The model under review builds one solid part; all positions refer to its coordinate system, in mm. Face numbers are marked on the shaded views. A direction names the side the tool comes from. Round coordinates to 2 decimals unless told otherwise and drop trailing zeros. Order: outer loops, then holes, each group sorted by start corner. A loop starts at its lowest first (then second) coordinate and runs counter-clockwise, first axis right, second up. Notation, with made-up numbers: M 55,52.5 L 68,52.5 A32 ccw 68,81.5 Z; hole C 54,-9.75 d9. An arc over 180 degrees is marked long. One line per item, written item: value. Start each with the question number.
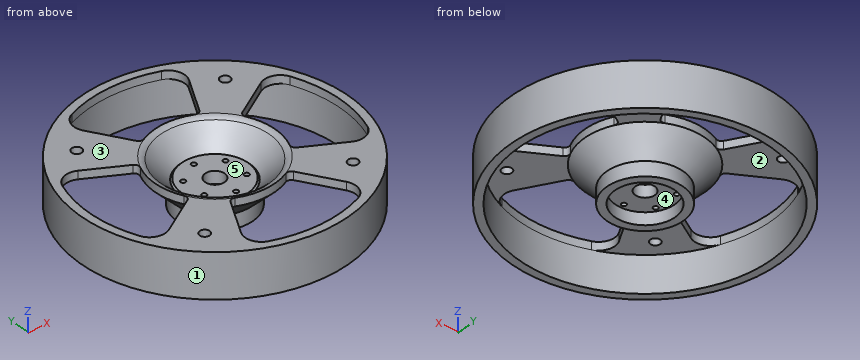
from build123d import *

# Parameters (mm, degrees)
EXTRUDE_1_DEPTH          = 20
EXTRUDE_1_DEPTH_BACK     = 7.5
SKETCH_1_R               = 82.5
SKETCH_1_R_2             = 80
EXTRUDE_3_DEPTH          = 7.5
EXTRUDE_3_DEPTH_BACK     = 7.5
SKETCH_3_R               = 21.5
CHAMFER_1_SIZE           = 1
SKETCH_4_R               = 18.5
CUT_EXTRUDE_1_DEPTH      = 7.5
SKETCH_5_R               = 1.5
CUT_EXTRUDE_2_DEPTH      = 7.5
SKETCH_6_R               = 6
CUT_EXTRUDE_3_DEPTH      = 7.5
SKETCH_9_R               = 3.1
CUT_EXTRUDE_4_DEPTH      = 119.822346
CUT_EXTRUDE_5_DEPTH      = 10
CUT_EXTRUDE_5_DEPTH_BACK = 119.822346


# Read off the part's stored shape, not the designer's step: the shell step
with BuildPart() as part:
    # Sketch 1 → Extrude 1 (new, two sides: drawn at the far end of the back side and taken through both)
    with BuildSketch(Plane.XY.offset(-EXTRUDE_1_DEPTH_BACK)):
        Circle(SKETCH_1_R)
        Circle(SKETCH_1_R_2, mode=Mode.SUBTRACT)
    extrude(amount=EXTRUDE_1_DEPTH + EXTRUDE_1_DEPTH_BACK)



with BuildPart() as body_2:
    # Sketch 3 → Extrude 3 (new, two sides: drawn at the far end of the back side and taken through both)
    with BuildSketch(Plane.XY.offset(-EXTRUDE_3_DEPTH_BACK)):
        Circle(SKETCH_3_R)
    extrude(amount=EXTRUDE_3_DEPTH + EXTRUDE_3_DEPTH_BACK)

    # Chamfer 1
    chamfer_1_edges = [body_2.edges().sort_by_distance(p)[0] for p in [
        (-21.5, 0, 7.5),
    ]]
    chamfer(chamfer_1_edges, length=CHAMFER_1_SIZE)

    # Sketch 4 → Cut-Extrude 1 (cut)
    with BuildSketch(Plane(origin=(0, 0, -7.5), x_dir=(-1, 0, 0), z_dir=(0, 0, -1))):
        Circle(SKETCH_4_R)
    extrude(amount=-CUT_EXTRUDE_1_DEPTH, mode=Mode.SUBTRACT)

    # Sketch 5 → Cut-Extrude 2 (cut)
    with BuildSketch(Plane.XY.offset(7.5)):
        with Locations((0, 15.5)):
            Circle(SKETCH_5_R)
        with Locations((13.423394, 7.75)):
            Circle(SKETCH_5_R)
        with Locations((13.423394, -7.75)):
            Circle(SKETCH_5_R)
        with Locations((0, -15.5)):
            Circle(SKETCH_5_R)
        with Locations((-13.423394, -7.75)):
            Circle(SKETCH_5_R)
        with Locations((-13.423394, 7.75)):
            Circle(SKETCH_5_R)
    extrude(amount=-CUT_EXTRUDE_2_DEPTH, mode=Mode.SUBTRACT)

    # Sketch 6 → Cut-Extrude 3 (cut)
    with BuildSketch(Plane.XY.offset(7.5)):
        Circle(SKETCH_6_R)
    extrude(amount=-CUT_EXTRUDE_3_DEPTH, mode=Mode.SUBTRACT)


with BuildPart() as part_1:
    add(part.part)

    add(body_2.part)  # Revolve 1 merges body 2
    # Sketch 8 → Revolve 1 (revolve)
    with BuildSketch(Plane(origin=(0, 0, 0), x_dir=(1, 0, 0), z_dir=(0, 1, 0)), mode=Mode.PRIVATE) as revolve_1_sk:
        with BuildLine():
            Line((-37.071068, -20), (-80, -20))
            Line((-80, -20), (-80, 0))
            Line((-80, 0), (-80, 0.5))
            Line((-80, 0.5), (-80, 7.5))
            Line((-80, 7.5), (-21.5, 7.5))
            Line((-21.5, 7.5), (-21.5, -6.5))
            Line((-21.5, -6.5), (-33.535534, -18.535534))
            ThreePointArc((-33.535534, -18.535534), (-35.157651, -19.619398), (-37.071068, -20))
        make_face()
    revolve(revolve_1_sk.sketch.rotate(Axis((0, 0, 0), (0, 0, -1)), 180), axis=Axis((0, 0, 0), (0, 0, -1)))

    # Shell 1 outline → Shell 1 (revolve, cut)
    with BuildSketch(Plane.XZ):
        Polygon((37.071068, 15), (23.5, 1.428932), (23.5, -7.5), (77.5, -7.5), (77.5, 15), align=None)
    revolve(axis=Axis((0, 0, 0), (0, 0, 1)), mode=Mode.SUBTRACT)

    # Sketch 9 → Cut-Extrude 4 (cut, through all)
    with BuildSketch(Plane(origin=(0, 0, 15), x_dir=(-1, 0, 0), z_dir=(0, 0, -1))):
        with Locations((-46.97, 46.97)):
            Circle(SKETCH_9_R)
        with Locations((46.97, 46.97)):
            Circle(SKETCH_9_R)
        with Locations((46.97, -46.97)):
            Circle(SKETCH_9_R)
        with Locations((-46.97, -46.97)):
            Circle(SKETCH_9_R)
    extrude(amount=-CUT_EXTRUDE_4_DEPTH, mode=Mode.SUBTRACT)

    # Sketch 10 → Cut-Extrude 5 (cut, two sides: drawn at the far end of the back side and taken through both)
    with BuildSketch(Plane(origin=(0, 0, 15), x_dir=(-1, 0, 0), z_dir=(0, 0, -1)).offset(-CUT_EXTRUDE_5_DEPTH_BACK)):
        with BuildLine():
            Line((-33.377575, 57.811655), (-19.979305, 34.605171))
            ThreePointArc((-19.979305, 34.605171), (-18.265691, 33.238513), (-16.079948, 33.402086))
            ThreePointArc((-16.079948, 33.402086), (0, 37.071068), (16.079948, 33.402086))
            ThreePointArc((16.079948, 33.402086), (18.265691, 33.238513), (19.979305, 34.605171))
            Line((19.979305, 34.605171), (33.377575, 57.811655))
            ThreePointArc((33.377575, 57.811655), (34.157646, 66.110179), (28.379146, 72.117086))
            ThreePointArc((28.379146, 72.117086), (0, 77.5), (-28.379146, 72.117086))
            ThreePointArc((-28.379146, 72.117086), (-34.157646, 66.110179), (-33.377575, 57.811655))
        make_face()
        with BuildLine():
            Line((57.811655, 33.377575), (34.605171, 19.979305))
            ThreePointArc((34.605171, 19.979305), (33.238513, 18.265691), (33.402086, 16.079948))
            ThreePointArc((33.402086, 16.079948), (37.071068, 0), (33.402086, -16.079948))
            ThreePointArc((33.402086, -16.079948), (33.238513, -18.265691), (34.605171, -19.979305))
            Line((34.605171, -19.979305), (57.811655, -33.377575))
            ThreePointArc((57.811655, -33.377575), (66.110179, -34.157646), (72.117086, -28.379146))
            ThreePointArc((72.117086, -28.379146), (77.5, 0), (72.117086, 28.379146))
            ThreePointArc((72.117086, 28.379146), (66.110179, 34.157646), (57.811655, 33.377575))
        make_face()
        with BuildLine():
            Line((33.377575, -57.811655), (19.979305, -34.605171))
            ThreePointArc((19.979305, -34.605171), (18.265691, -33.238513), (16.079948, -33.402086))
            ThreePointArc((16.079948, -33.402086), (0, -37.071068), (-16.079948, -33.402086))
            ThreePointArc((-16.079948, -33.402086), (-18.265691, -33.238513), (-19.979305, -34.605171))
            Line((-19.979305, -34.605171), (-33.377575, -57.811655))
            ThreePointArc((-33.377575, -57.811655), (-34.157646, -66.110179), (-28.379146, -72.117086))
            ThreePointArc((-28.379146, -72.117086), (0, -77.5), (28.379146, -72.117086))
            ThreePointArc((28.379146, -72.117086), (34.157646, -66.110179), (33.377575, -57.811655))
        make_face()
        with BuildLine():
            Line((-57.811655, -33.377575), (-34.605171, -19.979305))
            ThreePointArc((-34.605171, -19.979305), (-33.238513, -18.265691), (-33.402086, -16.079948))
            ThreePointArc((-33.402086, -16.079948), (-37.071068, 0), (-33.402086, 16.079948))
            ThreePointArc((-33.402086, 16.079948), (-33.238513, 18.265691), (-34.605171, 19.979305))
            Line((-34.605171, 19.979305), (-57.811655, 33.377575))
            ThreePointArc((-57.811655, 33.377575), (-66.110179, 34.157646), (-72.117086, 28.379146))
            ThreePointArc((-72.117086, 28.379146), (-77.5, 0), (-72.117086, -28.379146))
            ThreePointArc((-72.117086, -28.379146), (-66.110179, -34.157646), (-57.811655, -33.377575))
        make_face()
    extrude(amount=CUT_EXTRUDE_5_DEPTH + CUT_EXTRUDE_5_DEPTH_BACK, mode=Mode.SUBTRACT)


solid = part_1.part
Item 1: Consider section B-B, the plane x = -47.5. Give the boundary of the cut face in (y, z), then the cut area to 3 significant figures.
Item 2: The part is to be moulded in two halves that separate along X. For the marked faces 1, 2 and 3, say which applies: pulls with the +X half, pulls with the -X half, needs draft (parallel to the pull), parting line crosses it, or undercut.
Item 3: Wall thickness on L1, parallel to Y at x = 0, z = 4.25; L2, parallel to Y at x = 3, z = 11; L3, parallel to Y at x = -46.97, z = 19.05: over which ranges is each line inside the solid? List them lowest first.
Item 4: Clearance check with flat-ended pins moving along their axes: P1, Ø4, axis at x = -19, z = 0.5, coming from the +Y side; P2, Ø1.5, axis at x = 53, z = 9, coming from the +Y side (3 decimals); P3, Ø8, axis at y = 24.5, z = 3, coming from the +X side. State where each tip first meets the part, or that it passes through.
Item 5: Consider section C-C, the plane x = 39.5. Give the boundary of the cut face in (y, z), then the cut area to 3 significant figures.
Item 6: Machinability: for the marked faces 4 and 5, which of the approach directions +Z, -Z, +X, -X, +Y, -Y give a long, thin tool a straight path to every point of the face, cutting with its end or side? Answer none if there is none.
Item 7: Consider section A-A, the plane y = 0. Count the separate pieces of the cut face and the enclosed holes in it, then the cut area to 3 significant figures.
Computed:
1. outline: M -67.45,-7.5 L -61.24,-7.5 L -61.24,15 L -50.02,15 L -50.02,20 L -67.45,20 Z; M -43.92,15 L -27.42,15 L -27.42,20 L -43.92,20 Z; M 27.42,15 L 43.92,15 L 43.92,20 L 27.42,20 Z; M 50.02,15 L 61.24,15 L 61.24,-7.5 L 67.45,-7.5 L 67.45,20 L 50.02,20 Z
1. area: 619 mm^2
2. face 1: parting line crosses it
2. face 2: undercut
2. face 3: needs draft
3. L1: y = -82.5 to -77.5, -26.32 to -17, -14 to -6, 6 to 14, 17 to 26.32, 77.5 to 82.5
3. L2: y = -82.45 to -77.44, -32.93 to -25.83, 25.83 to 32.93, 77.44 to 82.45
3. L3: y = -67.82 to -50.07, -43.87 to -27.12, 27.12 to 43.87, 50.07 to 67.82
4. P1: stops at y = 80.73
4. P2: stops at y = 63.845
4. P3: stops at x = 79.91
5. outline: M -72.43,-7.5 L -66.68,-7.5 L -66.68,15 L -22.81,15 L -22.81,20 L -72.43,20 Z; M 22.81,15 L 66.68,15 L 66.68,-7.5 L 72.43,-7.5 L 72.43,20 L 22.81,20 Z
5. area: 755 mm^2
6. face 4: -Z
6. face 5: +Z
7. separate pieces: 4
7. enclosed holes: 0
7. area: 798 mm^2
